```python
from build123d import *

# Parameters (mm, degrees)
SKETCH1_W           = 20
SKETCH1_H           = 20
SKETCH1_W_2         = 15
SKETCH1_H_2         = 15
BOSS_EXTRUDE1_DEPTH = 10
SKETCH2_R           = 1.5
CUT_EXTRUDE1_DEPTH  = 25.494897428
SKETCH3_R           = 1
CUT_EXTRUDE2_DEPTH  = 6


with BuildPart() as part:
    # Sketch1 → Boss-Extrude1 (new body)
    with BuildSketch(Plane(origin=(0, 0, 0), x_dir=(1, 0, 0), z_dir=(0, 1, 0))):
        Rectangle(SKETCH1_W, SKETCH1_H)
        Rectangle(SKETCH1_W_2, SKETCH1_H_2, mode=Mode.SUBTRACT)
    extrude(amount=BOSS_EXTRUDE1_DEPTH)

    # Sketch2 → Cut-Extrude1 (cut, through all)
    with BuildSketch(Plane.ZY.offset(10)):
        with Locations((0, 5)):
            Circle(SKETCH2_R)
    extrude(amount=-CUT_EXTRUDE1_DEPTH, mode=Mode.SUBTRACT)

    # Sketch3 → Cut-Extrude2 (cut)
    with BuildSketch(Plane(origin=(0, 10, 0), x_dir=(1, 0, 0), z_dir=(0, 1, 0))):
        with Locations(Location((-8.5, 8.5, 0), (0, 0, 270))):
            Circle(SKETCH3_R)
        with Locations(Location((8.5, 8.5, 0), (0, 0, 270))):
            Circle(SKETCH3_R)
        with Locations(Location((8.5, -8.5, 0), (0, 0, 270))):
            Circle(SKETCH3_R)
        with Locations(Location((-8.5, -8.5, 0), (0, 0, 270))):
            Circle(SKETCH3_R)
    extrude(amount=-CUT_EXTRUDE2_DEPTH, mode=Mode.SUBTRACT)


solid = part.part
```
CAD build for the part. Positions are in the model's coordinates, mm. A direction names the side the tool comes from. Round coordinates to 2 decimals unless told otherwise and drop trailing zeros. Write each loop counter-clockwise with the first axis right and the second up, starting at its lowest first coordinate (ties: lowest second). Pieces come first, ordered by that corner, then holes. Notation, with made-up numbers: (38.5, -20) - (91.5, -20) arc R28 ccw to (91.5, 17) - close; hole circle Ø9 at (15, 88). An arc over 180 degrees is marked (long way). Write item = value, one per line. Start each with the question number.
Q1. Band-saw the part on D-D (z = 4.25). Give the cut face in (x, y).
Q2. Drop a flat-ended pin along its axis: pin 1 (1.6 mm diameter, centred on x = 8.5, z = -8.5, fed in from +Y). Give the stop position or say it passes through.
Q3. Band-saw the part on C-C (x = -8.5). Give the cut face in (y, z).
Q4. Band-saw the part on A-A (z = 0). Give the cut face in (x, y), then the cut area to 3 significant figures.
Q5. Mould opens along Z. For faces 1 (the cylindrical face through (-8.77, 5.07, -1.5)), 2 (the flat face through (0, 5, -10)), 3 (the flat face through (-10, 3, 0)), 4 (the flat face through (-8, 4, 8)) say: pulls with the +Z half, pulls with the -Z half, needs draft (parallel to the pull), parting line crosses it, or undercut.
Q6. Probe L1, parallel to X at y = 6.6, z = 8.5; L2, parallel to Z at x = 1.5, y = 5.5. List the from-to ranges inside material, lowest first. Write a range as from..to.
Q7. Band-saw the part on B-B (y = 5). Give the cut face in (x, z).
Q8. Which spindle directions (+Z, -Z, +X, -X, +Y, -Y) get a long thin tool onto all of the face, cutting with end or side? Do faces 5 (the flat face through (-9, 0, 0)), 6 (the flat face through (-7.5, 5, 2)), 7 (the flat face through (9, 4, 8)). Say none if no direction does.
Answers below:
q1.outline = (-10, 0) - (-7.5, 0) - (-7.5, 10) - (-10, 10) - close; (7.5, 0) - (10, 0) - (10, 10) - (7.5, 10) - close
q2.pin_1 = 4
q3.outline = (0, -10) - (10, -10) - (10, -9.5) - (4, -9.5) - (4, -7.5) - (10, -7.5) - (10, 7.5) - (4, 7.5) - (4, 9.5) - (10, 9.5) - (10, 10) - (0, 10) - close; hole circle Ø3 at (5, 0)
q4.outline = (-10, 0) - (-7.5, 0) - (-7.5, 3.5) - (-10, 3.5) - close; (-10, 6.5) - (-7.5, 6.5) - (-7.5, 10) - (-10, 10) - close; (7.5, 0) - (10, 0) - (10, 3.5) - (7.5, 3.5) - close; (7.5, 6.5) - (10, 6.5) - (10, 10) - (7.5, 10) - close
q4.area = 35.0 mm2
q5.face_1 = undercut
q5.face_2 = pulls with the -Z half
q5.face_3 = needs draft
q5.face_4 = undercut
q6.L1 = -10..-9.5, -7.5..7.5, 9.5..10
q6.L2 = -10..-7.5, 7.5..10
q7.outline = (-10, -10) - (10, -10) - (10, -1.5) - (7.5, -1.5) - (7.5, -7.5) - (-7.5, -7.5) - (-7.5, -1.5) - (-10, -1.5) - close; (-10, 1.5) - (-7.5, 1.5) - (-7.5, 7.5) - (7.5, 7.5) - (7.5, 1.5) - (10, 1.5) - (10, 10) - (-10, 10) - close; hole circle Ø2 at (-8.5, -8.5); hole circle Ø2 at (-8.5, 8.5); hole circle Ø2 at (8.5, -8.5); hole circle Ø2 at (8.5, 8.5)
q8.face_5 = +Z, -Z, +X, -X, -Y
q8.face_6 = +Y, -Y
q8.face_7 = +Y
